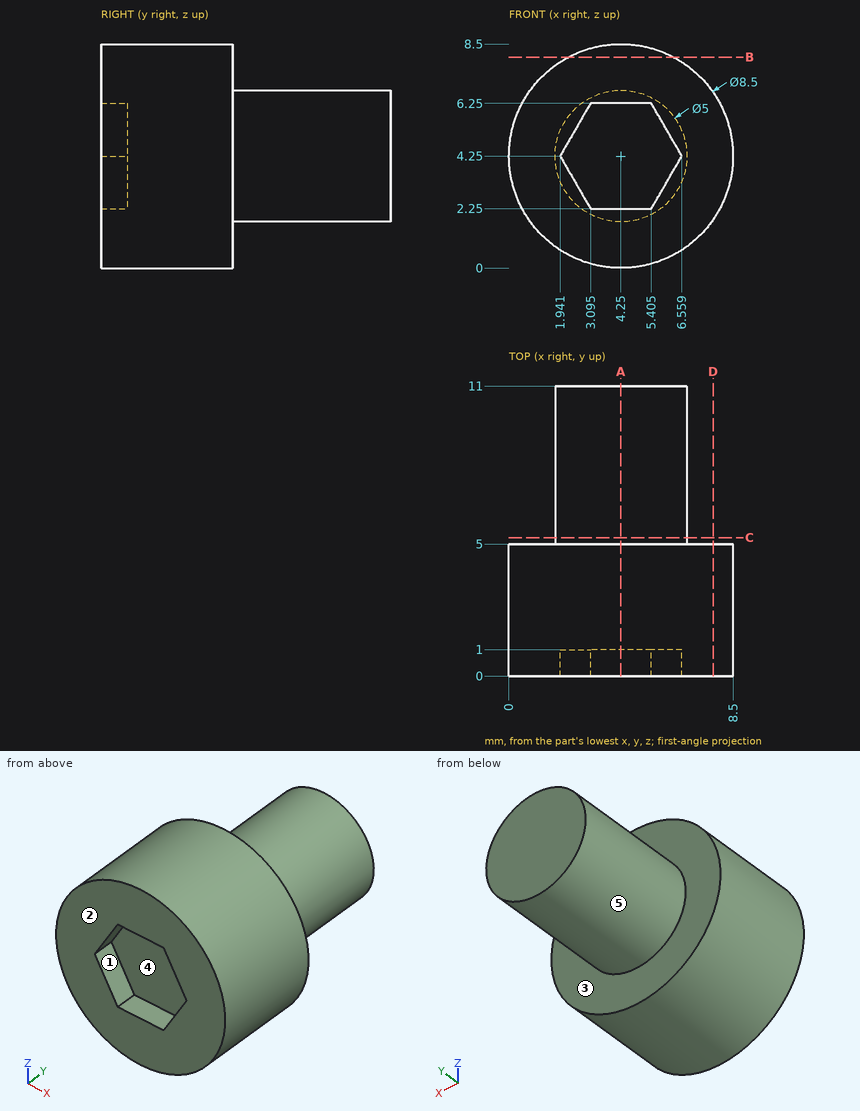
Source: three-view drawing plus pictorial views. Frame: mm from the lowest corner of the part. A direction names the side the tool comes from. Give positions to 0.01 mm unless a question says otherwise; leave off trailing zeros. Loops run counter-clockwise (first coordinate to the right, second up) from the corner with the lowest first, then second, coordinate; pieces in that order, holes last. Notation, with made-up numbers: (75, 68) -> (133, 68) arc R20 ccw to (133, 76) -> close; hole circle Ø5 at (80.5, -15.75). An arc over 180 degrees is marked (long way). Use a Markdown table: item, result. Add a question column.
(1) Pull-direction query (Z, two-part tool) for the marked faces 3, 4 and 5; classes: +Z half, -Z half, draft (parallel to the pull), parting line (faces both ways), or undercut.
(2) Section query A-A (x = 4.25). Output: boundary loops of the cut face in (y, z), then the cut area to 3 significant figures.
(3) Access query for the marked faces 1 and 2. Directions: +Z, -Z, +X, -X, +Y, -Y. A direction counts if a zero-diameter tool reaches every point of the face in a straight line with its end or side. Return the directions, or none.
(4) Ray query, line 1 (Y direction, x = 1.25, z = 3.75); line 2 (X direction, y = 2, z = 5.5); line 3 (Z direction, x = 3.25, y = 4.75). Return the intervals inside material, ascending.
(5) First-contact query: pin 1 Ø4 at (x, y) = (6, 7.5) entering from -Z; pin 2 Ø3 at (x, z) = (4, 4) entering from -Y; pin 3 Ø5 at (y, z) = (6, 5.5) entering from +X; pin 4 Ø1 at (x, y) = (7, 4.5) entering from +Z (1 decimal). Flat tips, straight axial feed; report the tip coordinate or a pass-through.
(6) Section query C-C (y = 5.25). Output: boundary loops of the cut face in (x, z).
(7) Section query D-D (x = 7.75). Output: boundary loops of the cut face in (y, z), then the cut area to 3 significant figures.
(8) Section query B-B (z = 8). Output: boundary loops of the cut face in (x, y).
Checked values:
| question | item | result |
|---|---|---|
| 1 | face 3 | draft |
| 1 | face 4 | undercut |
| 1 | face 5 | parting line |
| 2 | outline | (0, 0) -> (5, 0) -> (5, 1.75) -> (11, 1.75) -> (11, 6.75) -> (5, 6.75) -> (5, 8.5) -> (0, 8.5) -> (0, 6.25) -> (1, 6.25) -> (1, 2.25) -> (0, 2.25) -> close |
| 2 | area | 68.5 mm^2 |
| 3 | face 1 | -Y |
| 3 | face 2 | +Z, -Z, +X, -X, -Y |
| 4 | line 1 | 0 to 5 |
| 4 | line 2 | 0.19 to 8.31 |
| 4 | line 3 | 0.12 to 8.38 |
| 5 | pin 1 | z = 1.75 |
| 5 | pin 2 | y = 1 |
| 5 | pin 3 | x = 8.5 |
| 5 | pin 4 | z = 7.9 |
| 6 | outline | circle Ø5 at (4.25, 4.25) |
| 7 | outline | (0, 1.84) -> (5, 1.84) -> (5, 6.66) -> (0, 6.66) -> close |
| 7 | area | 24.1 mm^2 |
| 8 | outline | (2.25, 0) -> (6.25, 0) -> (6.25, 5) -> (2.25, 5) -> close |
